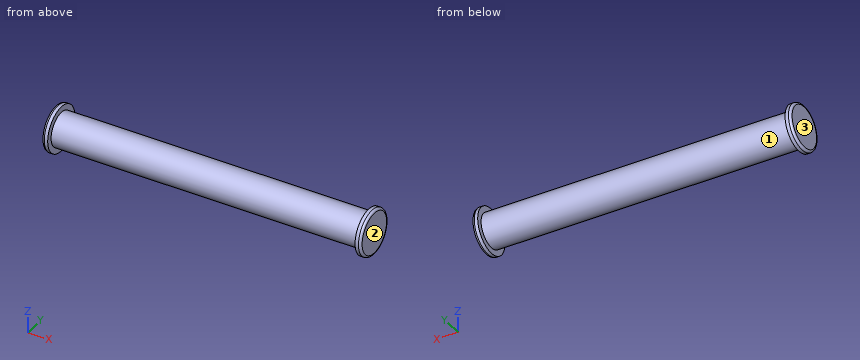
```python
from build123d import *

# Parameters (mm, degrees)
SKETCH1_R           = 1.5
BOSS_EXTRUDE1_DEPTH = 13.5
SKETCH2_R           = 2
BOSS_EXTRUDE2_DEPTH = 0.5
SKETCH3_R           = 2
BOSS_EXTRUDE3_DEPTH = 0.5
FILLET1_R           = 0.2


with BuildPart() as part:
    # Sketch1 → Boss-Extrude1 (new body, symmetric)
    with BuildSketch(Plane(origin=(0, 0, 0), x_dir=(0, 0, -1), z_dir=(1, 0, 0))):
        Circle(SKETCH1_R)
    extrude(amount=BOSS_EXTRUDE1_DEPTH, both=True)

    # Sketch2 → Boss-Extrude2 (add)
    with BuildSketch(Plane(origin=(13.5, 0, 0), x_dir=(0, 0, -1), z_dir=(1, 0, 0))):
        Circle(SKETCH2_R)
    extrude(amount=BOSS_EXTRUDE2_DEPTH)

    # Sketch3 → Boss-Extrude3 (add)
    with BuildSketch(Plane.ZY.offset(13.5)):
        Circle(SKETCH3_R)
    extrude(amount=BOSS_EXTRUDE3_DEPTH)

    # Fillet1
    fillet1_edges = [part.edges().sort_by_distance(p)[0] for p in [
        (-14, 0, -2),
        (14, 0, 2),
    ]]
    fillet(fillet1_edges, radius=FILLET1_R)


solid = part.part
```
Check sheet for the modelled part. Datum: model origin and axes. Units: mm. Face numbers are marked on the shaded views. Coordinates: 2 decimals unless noted, no trailing zeros. Loops run counter-clockwise (first coordinate to the right, second up) from the corner with the lowest first, then second, coordinate; pieces in that order, holes last.
1) Release check for a two-part mould opening along X. For the marked faces 1, 2 and 3 record: released by +X, released by -X, zero draft, split by the parting line, or undercut.
2) Sectioned sample at C-C (x = 6.75). Record the boundary of the cut face in (y, z), and give its area (3 significant figures).
3) Material ranges on probe 1 along X at (y, z) = (0.4, 1.5); probe 2 along Y at (x, z) = (2.5, 0), recorded low to high.
4) Sectioned sample at A-A (y = 0). Record the boundary of the cut face in (x, z), and give its area (3 significant figures).
Check sheet entries:
1. face 1: undercut
1. face 2: released by +X
1. face 3: released by -X
2. outline: circle Ø3 at (0, 0)
2. area: 7.07 mm2
3. probe 1: x = -14 to -13.5, 13.5 to 14
3. probe 2: y = -1.5 to 1.5
4. outline: (-14, -1.8) arc R0.2 ccw to (-13.8, -2) - (-13.5, -2) - (-13.5, -1.5) - (13.5, -1.5) - (13.5, -2) - (13.8, -2) arc R0.2 ccw to (14, -1.8) - (14, 1.8) arc R0.2 ccw to (13.8, 2) - (13.5, 2) - (13.5, 1.5) - (-13.5, 1.5) - (-13.5, 2) - (-13.8, 2) arc R0.2 ccw to (-14, 1.8) - close
4. area: 85.0 mm2
